Could you check a few things on this model? Use its own coordinates, in mm. Face numbers are marked on the shaded views. A direction names the side the tool comes from. Coordinates: 2 decimals unless noted, no trailing zeros. Loops run counter-clockwise (first coordinate to the right, second up) from the corner with the lowest first, then second, coordinate; pieces in that order, holes last. Notation, with made-up numbers: (-30.5, 19) - (8.5, 19) arc R17 cw to (8.5, 51) - close; hole circle Ø8 at (24.25, 3.5). An arc over 180 degrees is marked (long way). One line per question, with ' | ' between items. Start each with the question number.
1. I want a section at C-C, the plane z = -28.5. Write out the boundary of the cut face in (x, y), then the cut area to 3 significant figures.
2. I'm going to push flat-ended pins straight in: P1, Ø12, axis at x = 14.5, z = 1, coming from the +Y side; P2, Ø7, axis at y = -112.5, z = 0, coming from the -X side; P3, Ø15, axis at x = 28, y = -113, coming from the +Z side. Where does each tip first touch, or does it pass through?
3. I want a section at D-D, the plane x = 15. Write out the boundary of the cut face in (y, z).
4. I want a section at B-B, the plane y = -67. Write out the boundary of the cut face in (x, z).
5. Please list where these lines run through material, in increasing order: L1, parallel to X at y = -33, z = 0.5; L2, parallel to X at y = 27.5, z = -16; L3, parallel to Z at x = 27, y = -171. Write a range as [from, to].
6. I want a section at A-A, the plane x = 25.5. Write out the boundary of the cut face in (y, z).
7. Which directions (+Z, -Z, +X, -X, +Y, -Y) give clear straight access to the entire face, cutting with the end or side of a thin tool? Please do the marked faces 1, 2 and 3.
from build123d import *

# Parameters (mm, degrees)
F0_R     = 64.5
F1_DEPTH = 3
F2_R     = 12
F3_DEPTH = 19
F5_DEPTH = 19.05


with BuildPart() as f1:
    # F0 (on Right) → F1 (new body)
    with BuildSketch(Plane.YZ):
        Circle(F0_R)
    extrude(amount=F1_DEPTH)

    # F2 (on face) → F3 (join)
    with BuildSketch(Plane.YZ.offset(3)):
        Circle(F2_R)
    extrude(amount=F3_DEPTH)

    # F4 (on face) → F5 (join)
    with BuildSketch(Plane.YZ.offset(22)):
        with BuildLine():
            ThreePointArc((0, -12), (-12, 0), (0, 12))
            Line((0, 12), (-180, 12))
            ThreePointArc((-180, 12), (-192, 0), (-180, -12))
            Line((-180, -12), (0, -12))
        make_face()
        with BuildLine():
            ThreePointArc((12, 0), (8.485281, 8.485281), (0, 12))
            ThreePointArc((0, 12), (-12, 0), (0, -12))
            ThreePointArc((0, -12), (8.485281, -8.485281), (12, 0))
        make_face()
    extrude(amount=F5_DEPTH)


solid = f1.part
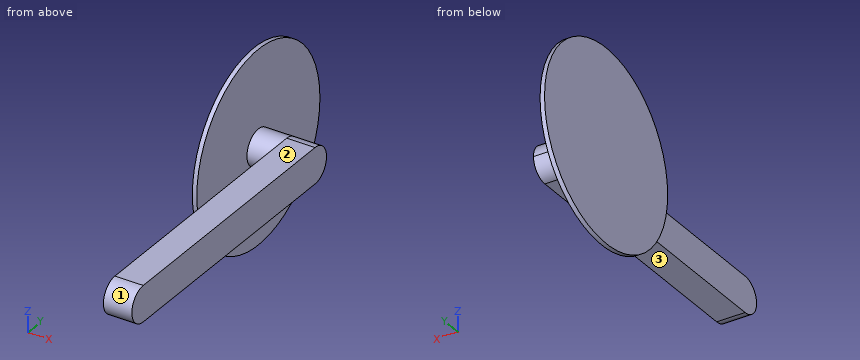
Results are:
1) outline: (0, -57.86) - (3, -57.86) - (3, 57.86) - (0, 57.86) - close | area: 347 mm2
2) P1: stops at y = 12 | P2: stops at x = 22 | P3: stops at z = 12
3) outline: circle Ø24 at (0, 0)
4) outline: (22, -12) - (41.05, -12) - (41.05, 12) - (22, 12) - close
5) L1: x = [0, 3], [22, 41.05] | L2: x = [0, 3] | L3: z = [-12, 12]
6) outline: (-180, -12) - (0, -12) arc R12 ccw to (12, 0) arc R12 ccw to (0, 12) - (-180, 12) arc R12 ccw to start
7) face 1: +X, -X, -Y | face 2: +Z, +X, +Y, -Y | face 3: -Z, +X, +Y, -Y
